from build123d import *

# Parameters (mm, degrees)
F0_R     = 190.5
F2_DEPTH = 762
F0_W     = 177.8
F0_H     = 1066.8
F3_DEPTH = 228.6
F4_DEPTH = 88.9
F5_DEPTH = 88.9


with BuildPart() as f2:
    # F0 (on Top) → F2 (new body)
    with BuildSketch(Plane.XY):
        with BuildLine():
            Line((88.9, -131.90195), (381, -131.90195))
            Line((381, -131.90195), (381, 325.29805))
            ThreePointArc((381, 325.29805), (0, 706.29805), (-381, 325.29805))
            Line((-381, 325.29805), (-381, -131.90195))
            Line((-381, -131.90195), (-88.9, -131.90195))
            Line((-88.9, -131.90195), (88.9, -131.90195))
        make_face()
        with Locations((0, 325.29805)):
            Circle(F0_R, mode=Mode.SUBTRACT)
    extrude(amount=F2_DEPTH)

    # F0 (on Top) → F3 (join)
    with BuildSketch(Plane.XY):
        Polygon((381, -970.10195), (381, -131.90195), (88.9, -131.90195), (88.9, -1198.70195), align=None)
        with BuildLine():
            Line((88.9, -131.90195), (381, -131.90195))
            Line((381, -131.90195), (381, 325.29805))
            ThreePointArc((381, 325.29805), (0, 706.29805), (-381, 325.29805))
            Line((-381, 325.29805), (-381, -131.90195))
            Line((-381, -131.90195), (-88.9, -131.90195))
            Line((-88.9, -131.90195), (88.9, -131.90195))
        make_face()
        with Locations((0, 325.29805)):
            Circle(F0_R, mode=Mode.SUBTRACT)
        with Locations((0, -665.30195)):
            Rectangle(F0_W, F0_H)
        Polygon((-88.9, -1198.70195), (-88.9, -131.90195), (-381, -131.90195), (-381, -970.10195), align=None)
    extrude(amount=F3_DEPTH)

    # F1 (on Right) → F4 (join)
    with BuildSketch(Plane.YZ):
        Polygon((-129.027212, 762), (-1196.931251, 228.6), (-977.461457, 228.6), (-129.027212, 228.6), align=None)
    extrude(amount=F4_DEPTH)

    # F4_face (on face) → F5 (join)
    with BuildSketch(Plane(origin=(0, -486.911717, 405.921372), x_dir=(0, 1, 0), z_dir=(-1, 0, 0))):
        Polygon((-710.019534, 177.321372), (355.009767, -354.642745), (355.009767, 177.321372), align=None)
    extrude(amount=F5_DEPTH)


solid = f2.part
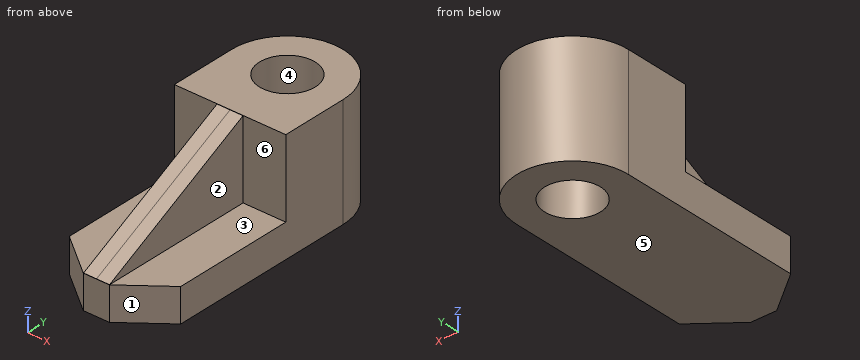
The model under review builds one solid part; all positions refer to its coordinate system, in mm. Face numbers are marked on the shaded views. A direction names the side the tool comes from. Give positions to 0.01 mm unless a question says otherwise; leave off trailing zeros. Loops run counter-clockwise (first coordinate to the right, second up) from the corner with the lowest first, then second, coordinate; pieces in that order, holes last. Notation, with made-up numbers: (36, 10.5) -> (48, 10.5) arc R8 cw to (48, 16.5) -> close; hole circle Ø2 at (11, 54.5). An arc over 180 degrees is marked (long way). Answer as a JSON object with one key per item and string values. Group by question number.
Q1. Take a section at D-D (z = 273.5). Write out the cut boundary in (x, y), plus the area to 3 significant figures.
Q2. Take a section at A-A (z = 187.5). Write out the cut boundary in (x, y), plus the area to 3 significant figures.
Q3. Draft analysis for pull direction Y (two halves, no side actions). For the marked faces 4, 5 and 6, state which applies: pulls with the +Y half, pulls with the -Y half, needs draft (parallel to the pull), parting line crosses it, or undercut.
Q4. Insertion check: pin 1 (1 mm diameter, centred on x = 89.5, z = 277.5, fed in from -Y); pin 2 (1.5 mm diameter, centred on x = 204, z = 621.5, fed in from +Y); pin 3 (4 mm diameter, centred on x = -56, z = 408, fed in from -Y). Each pin has a flat end and moves straight along its axis. Give the tip position at first contact, or say it passes through.
Q5. Take a section at B-B (x = -37.5). Write out the cut boundary in (y, z), plus the area to 3 significant figures.
Q6. Wall thickness on line 1 along Y through (x, z) = (0, 174.5); line 2 along X through (y, z) = (-199, 530); line 3 along Z through (x, y) = (115, -290): over which ranges is each line inside the solid? List them lowest first.
Q7. Take a section at C-C (y = 212.5). Write out the cut boundary in (x, z).
Q8. Tool access review of the marked faces 1, 2 and 3: name each direction out of +Z, -Z, +X, -X, +Y, -Y from which nothing blocks a thin tool from reaching the whole face with its end or side.
Answer below:
{
 "1": {"outline": "(-381, -131.9) -> (-88.9, -131.9) -> (-88.9, -1107.04) -> (88.9, -1107.04) -> (88.9, -131.9) -> (381, -131.9) -> (381, 325.3) arc R381 ccw to (-381, 325.3) -> close; hole circle Ø381 at (0, 325.3)", "area": "636,000 mm2"},
 "2": {"outline": "(-381, -970.1) -> (-88.9, -1198.7) -> (88.9, -1198.7) -> (381, -970.1) -> (381, 325.3) arc R381 ccw to (-381, 325.3) -> close; hole circle Ø381 at (0, 325.3)", "area": "1,210,000 mm2"},
 "3": {"face 4": "undercut", "face 5": "needs draft", "face 6": "pulls with the -Y half"},
 "4": {"pin 1": "stops at y = -131.9", "pin 2": "stops at y = 647.56", "pin 3": "stops at y = -841.76"},
 "5": {"outline": "(-1198.7, 0) -> (138.53, 0) -> (138.53, 762) -> (-131.9, 762) -> (-131.9, 760.56) -> (-1196.93, 228.6) -> (-1198.7, 228.6) -> close; (512.07, 0) -> (704.45, 0) -> (704.45, 762) -> (512.07, 762) -> close", "area": "880,000 mm2"},
 "6": {"line 1": "y = -1198.7 to 134.8, 515.8 to 706.3", "line 2": "x = -88.9 to 88.9", "line 3": "z = 0 to 228.6"},
 "7": {"outline": "(-381, 0) -> (-153.51, 0) -> (-153.51, 762) -> (-381, 762) -> close; (153.51, 0) -> (381, 0) -> (381, 762) -> (153.51, 762) -> close"},
 "8": {"face 1": "+Z, -Z, +X, -Y", "face 2": "+Z, +X, -Y", "face 3": "+Z, -Y"}
}
